Answer from the drawing. Dimensions are ordinates in mm from the lowest x, y and z of the part. Round coordinates to 2 decimals unless told otherwise and drop trailing zeros. Write each loop counter-clockwise with the first axis right and the second up, starting at its lowest first coordinate (ties: lowest second). Pieces come first, ordered by that corner, then holes. Notation, with made-up numbers: (42.5, 61.5) - (97.5, 61.5) arc R22 cw to (97.5, 82.5) - close; hole circle Ø3 at (12, 34). An arc over 180 degrees is marked (long way). Answer in a Markdown table with one row per item.
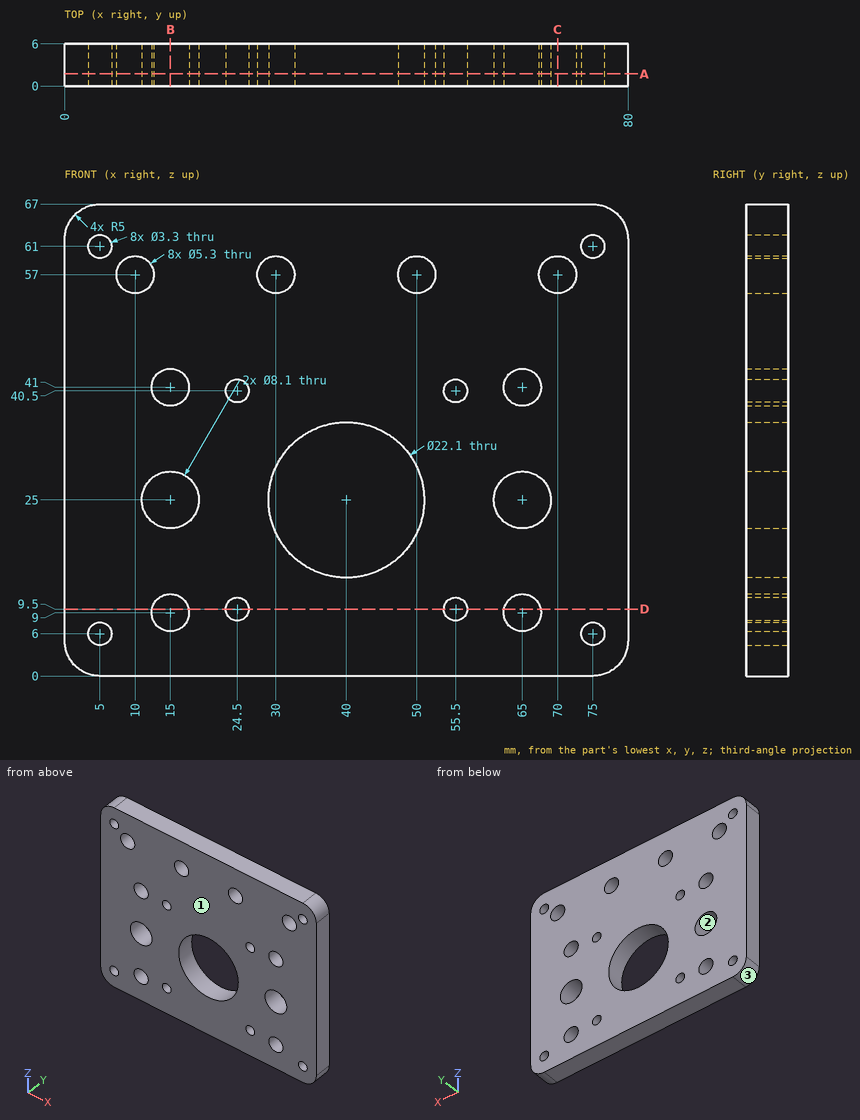
(1) Find the intervals of material crossed by line 1 (X direction, y = 2.7, z = 57); line 2 (Z direction, x = 65, y = 3.25); line 3 (Z direction, x = 75, y = 1.35), in increasing order.
Checked values:
| item | result |
|---|---|
| line 1 | x = 0 to 7.35, 12.65 to 27.35, 32.65 to 47.35, 52.65 to 67.35, 72.65 to 80 |
| line 2 | z = 0 to 6.35, 11.65 to 20.95, 29.05 to 38.35, 43.65 to 67 |
| line 3 | z = 0 to 4.35, 7.65 to 59.35, 62.65 to 67 |
(2) Section D-D (z = 9.5) is taken. Give the vertices of the cut face in (x, y), and give its area (3 significant figures).
Checked values:
| item | result |
|---|---|
| outline | (0, 0) - (12.4, 0) - (12.4, 6) - (0, 6) - close; (17.6, 0) - (22.85, 0) - (22.85, 6) - (17.6, 6) - close; (26.15, 0) - (53.85, 0) - (53.85, 6) - (26.15, 6) - close; (57.15, 0) - (62.4, 0) - (62.4, 6) - (57.15, 6) - close; (67.6, 0) - (80, 0) - (80, 6) - (67.6, 6) - close |
| area | 378 mm2 |
(3) Section B-B (x = 15) is taken. Give the vertices of the cut face in (y, z), and give its area (3 significant figures).
Checked values:
| item | result |
|---|---|
| outline | (0, 0) - (6, 0) - (6, 6.35) - (0, 6.35) - close; (0, 11.65) - (6, 11.65) - (6, 20.95) - (0, 20.95) - close; (0, 29.05) - (6, 29.05) - (6, 38.35) - (0, 38.35) - close; (0, 43.65) - (6, 43.65) - (6, 67) - (0, 67) - close |
| area | 290 mm2 |
(4) Section A-A (y = 1.75) is taken. State how many separate pieces and enclosed holes the cut face has, and give its area (3 significant figures).
Checked values:
| item | result |
|---|---|
| separate pieces | 1 |
| enclosed holes | 19 |
| area | 4,610 mm2 |
(5) A flat-ended cylindrical pin translates along its axis: pin 1 (5 mm diameter, centred on x = 15, z = 25, fed in from -Y). Find the tip coordinate at first contact, or state that the pin passes through.
Checked values:
| item | result |
|---|---|
| pin 1 | passes through |
(6) Section C-C (x = 70) is taken. Give the vertices of the cut face in (y, z).
Checked values:
| item | result |
|---|---|
| outline | (0, 0) - (6, 0) - (6, 54.35) - (0, 54.35) - close; (0, 59.65) - (6, 59.65) - (6, 67) - (0, 67) - close |
(7) For a pull along Z with two mould halves and no side action, classify the marked faces 1, 2 and 3 as pulls with the +Z half, pulls with the -Z half, needs draft (parallel to the pull), parting line crosses it, or undercut.
Checked values:
| item | result |
|---|---|
| face 1 | needs draft |
| face 2 | undercut |
| face 3 | pulls with the -Z half |
